Here's how the part is built. I have some questions about the finished solid (model axes, mm). A direction names the side the tool comes from. Coordinates: 2 decimals unless noted, no trailing zeros. Write each loop counter-clockwise with the first axis right and the second up, starting at its lowest first coordinate (ties: lowest second). Pieces come first, ordered by that corner, then holes. Notation, with made-up numbers: (34.5, 74.5) -> (77.5, 74.5) arc R17 cw to (77.5, 96.5) -> close; hole circle Ø2 at (67, -6). An arc over 180 degrees is marked (long way). Answer in a Markdown table with one row per item. Add a question column.
from build123d import *

# Parameters (mm, degrees)
F1_DEPTH  = 3.81
F4_DEPTH  = 71.628
F6_DEPTH  = 1.27
F7_W      = 13.462
F7_H      = 6.477
F8_DEPTH  = 25.4
F9_W      = 54.61
F9_H      = 4.318
F10_DEPTH = 25.4


with BuildPart() as f1:
    # F0 (on Front) → F1 (new body)
    with BuildSketch(Plane.XZ):
        Polygon((-38.4448663006, 16.8945933835), (-38.4448663006, 14.7355933835), (33.1831336994, 14.7355933835), (33.1831336994, 16.8945933835), (28.6111336994, 16.8945933835), (27.0871336994, 16.8945933835), (22.5151336994, 16.8945933835), (20.9911336994, 16.8945933835), (16.4191336994, 16.8945933835), (14.8951336994, 16.8945933835), (10.3231336994, 16.8945933835), (8.7991336994, 16.8945933835), (4.2271336994, 16.8945933835), (2.7031336994, 16.8945933835), (-1.8688663006, 16.8945933835), (-3.3928663006, 16.8945933835), (-7.9648663006, 16.8945933835), (-9.4888663006, 16.8945933835), (-14.0608663006, 16.8945933835), (-15.5848663006, 16.8945933835), (-20.1568663006, 16.8945933835), (-21.6808663006, 16.8945933835), (-26.2528663006, 16.8945933835), (-27.7768663006, 16.8945933835), (-32.3488663006, 16.8945933835), (-33.8728663006, 16.8945933835), align=None)
        Polygon((-37.1748663006, 21.2125933835), (-38.4448663006, 16.8945933835), (-33.8728663006, 16.8945933835), (-35.1428663006, 21.2125933835), align=None)
        Polygon((28.6111336994, 16.8945933835), (33.1831336994, 16.8945933835), (31.9131336994, 21.2125933835), (29.8811336994, 21.2125933835), align=None)
        Polygon((-31.0788663006, 21.2125933835), (-32.3488663006, 16.8945933835), (-27.7768663006, 16.8945933835), (-29.0468663006, 21.2125933835), align=None)
        Polygon((22.5151336994, 16.8945933835), (27.0871336994, 16.8945933835), (25.8171336994, 21.2125933835), (23.7851336994, 21.2125933835), align=None)
        Polygon((-24.9828663006, 21.2125933835), (-26.2528663006, 16.8945933835), (-21.6808663006, 16.8945933835), (-22.9508663006, 21.2125933835), align=None)
        Polygon((16.4191336994, 16.8945933835), (20.9911336994, 16.8945933835), (19.7211336994, 21.2125933835), (17.6891336994, 21.2125933835), align=None)
        Polygon((-18.8868663006, 21.2125933835), (-20.1568663006, 16.8945933835), (-15.5848663006, 16.8945933835), (-16.8548663006, 21.2125933835), align=None)
        Polygon((10.3231336994, 16.8945933835), (14.8951336994, 16.8945933835), (13.6251336994, 21.2125933835), (11.5931336994, 21.2125933835), align=None)
        Polygon((-12.7908663006, 21.2125933835), (-14.0608663006, 16.8945933835), (-9.4888663006, 16.8945933835), (-10.7588663006, 21.2125933835), align=None)
        Polygon((4.2271336994, 16.8945933835), (8.7991336994, 16.8945933835), (7.5291336994, 21.2125933835), (5.4971336994, 21.2125933835), align=None)
        Polygon((-6.6948663006, 21.2125933835), (-7.9648663006, 16.8945933835), (-3.3928663006, 16.8945933835), (-4.6628663006, 21.2125933835), align=None)
        Polygon((-1.8688663006, 16.8945933835), (2.7031336994, 16.8945933835), (1.4331336994, 21.2125933835), (-0.5988663006, 21.2125933835), align=None)
    extrude(amount=F1_DEPTH)

    # F3 (on plane+point) → F4 (join, through all)
    with BuildSketch(Plane.YZ.offset(33.1831336994)):
        Polygon((-13.97, 14.7355933835), (-3.81, 14.7355933835), (-3.81, 16.8945933835), (-10.16, 16.8945933835), (-10.16, 19.0535933835), (-13.97, 19.0535933835), (-13.97, 16.8945933835), align=None)
    extrude(amount=-F4_DEPTH)

    # F5 (on face) → F6 (join)
    with BuildSketch(Plane(origin=(0, 0, 0), x_dir=(-1, 0, 0), z_dir=(0, 1, 0))):
        Polygon((33.8728663006, 16.8945933835), (35.1428663006, 21.2125933835), (31.0788663006, 21.2125933835), (32.3488663006, 16.8945933835), align=None)
        Polygon((27.7768663006, 16.8945933835), (29.0468663006, 21.2125933835), (24.9828663006, 21.2125933835), (26.2528663006, 16.8945933835), align=None)
        Polygon((21.6808663006, 16.8945933835), (22.9508663006, 21.2125933835), (18.8868663006, 21.2125933835), (20.1568663006, 16.8945933835), align=None)
        Polygon((15.5848663006, 16.8945933835), (16.8548663006, 21.2125933835), (12.7908663006, 21.2125933835), (14.0608663006, 16.8945933835), align=None)
        Polygon((9.4888663006, 16.8945933835), (10.7588663006, 21.2125933835), (6.6948663006, 21.2125933835), (7.9648663006, 16.8945933835), align=None)
        Polygon((3.3928663006, 16.8945933835), (4.6628663006, 21.2125933835), (0.5988663006, 21.2125933835), (1.8688663006, 16.8945933835), align=None)
        Polygon((-1.4331336994, 21.2125933835), (-5.4971336994, 21.2125933835), (-4.2271336994, 16.8945933835), (-2.7031336994, 16.8945933835), align=None)
        Polygon((-7.5291336994, 21.2125933835), (-11.5931336994, 21.2125933835), (-10.3231336994, 16.8945933835), (-8.7991336994, 16.8945933835), align=None)
        Polygon((-13.6251336994, 21.2125933835), (-17.6891336994, 21.2125933835), (-16.4191336994, 16.8945933835), (-14.8951336994, 16.8945933835), align=None)
        Polygon((-19.7211336994, 21.2125933835), (-23.7851336994, 21.2125933835), (-22.5151336994, 16.8945933835), (-20.9911336994, 16.8945933835), align=None)
        Polygon((-25.8171336994, 21.2125933835), (-29.8811336994, 21.2125933835), (-28.6111336994, 16.8945933835), (-27.0871336994, 16.8945933835), align=None)
        Polygon((-33.1831336994, 14.7355933835), (38.4448663006, 14.7355933835), (38.4448663006, 16.8945933835), (37.1748663006, 21.2125933835), (35.1428663006, 21.2125933835), (33.8728663006, 16.8945933835), (32.3488663006, 16.8945933835), (31.0788663006, 21.2125933835), (29.0468663006, 21.2125933835), (27.7768663006, 16.8945933835), (26.2528663006, 16.8945933835), (24.9828663006, 21.2125933835), (22.9508663006, 21.2125933835), (21.6808663006, 16.8945933835), (20.1568663006, 16.8945933835), (18.8868663006, 21.2125933835), (16.8548663006, 21.2125933835), (15.5848663006, 16.8945933835), (14.0608663006, 16.8945933835), (12.7908663006, 21.2125933835), (10.7588663006, 21.2125933835), (9.4888663006, 16.8945933835), (7.9648663006, 16.8945933835), (6.6948663006, 21.2125933835), (4.6628663006, 21.2125933835), (3.3928663006, 16.8945933835), (1.8688663006, 16.8945933835), (0.5988663006, 21.2125933835), (-1.4331336994, 21.2125933835), (-2.7031336994, 16.8945933835), (-4.2271336994, 16.8945933835), (-5.4971336994, 21.2125933835), (-7.5291336994, 21.2125933835), (-8.7991336994, 16.8945933835), (-10.3231336994, 16.8945933835), (-11.5931336994, 21.2125933835), (-13.6251336994, 21.2125933835), (-14.8951336994, 16.8945933835), (-16.4191336994, 16.8945933835), (-17.6891336994, 21.2125933835), (-19.7211336994, 21.2125933835), (-20.9911336994, 16.8945933835), (-22.5151336994, 16.8945933835), (-23.7851336994, 21.2125933835), (-25.8171336994, 21.2125933835), (-27.0871336994, 16.8945933835), (-28.6111336994, 16.8945933835), (-29.8811336994, 21.2125933835), (-31.9131336994, 21.2125933835), (-33.1831336994, 16.8945933835), align=None)
        Polygon((37.1748663006, 21.2125933835), (38.4448663006, 16.8945933835), (38.4448663006, 21.2125933835), align=None)
    extrude(amount=F6_DEPTH)

    # F7 (on face) → F8 (join)
    with BuildSketch(Plane(origin=(0, 1.27, 0), x_dir=(-1, 0, 0), z_dir=(0, 1, 0))):
        with Locations((31.7138663006, 17.9740933835)):
            Rectangle(F7_W, F7_H)
    extrude(amount=F8_DEPTH)

    # F9 (on face) → F10 (cut)
    with BuildSketch(Plane.XY.offset(16.8945933835)):
        with Locations((-2.6308663007, -6.985)):
            Rectangle(F9_W, F9_H)
        with BuildLine():
            Line((24.6741336994, -4.826), (24.6741336994, -9.144))
            ThreePointArc((24.6741336994, -9.144), (26.8331336994, -6.985), (24.6741336994, -4.826))
        make_face()
        with BuildLine():
            ThreePointArc((-29.9358663007, -4.826), (-32.0948663007, -6.985), (-29.9358663007, -9.144))
            Line((-29.9358663007, -9.144), (-29.9358663007, -4.826))
        make_face()
    extrude(amount=-F10_DEPTH, mode=Mode.SUBTRACT)


solid = f1.part
Q1. For faces 3 (the flat face through (-28.4, -1.88, 19.02)), 4 (the flat face through (-3, -4.826, 16)), 5 (the flat face through (5, 1.27, 18)), which set-ups out of +Z, -Z, +X, -X, +Y, -Y let a thin tool reach every point of the face, with its end or its side?
Q2. Imagine slicing it at D-D on y = 11. Please give me the cut outline in (x, z), plus the area to 3 significant figures.
Q3. Imagine slicing it at C-C on y = -5.5. Please give me the cut outline in (x, z).
Q4. I'm going to push flat-ended pins straight in: P1, Ø1, axis at x = -10, z = 17.5, coming from the +Y side; P2, Ø1.9, axis at x = -6.5, y = -13, coming from the +Z side; P3, Ø3, axis at y = 10.5, z = 18.5, coming from the +X side; P4, Ø1, axis at x = -15.5, y = 3, coming from the -Z side. Where does each tip first touch, or does it pass through?
Q5. If we mould it in two halves opening along X, with no side actions, what happens to faces 1 (the flat face through (-7.321, -1.878, 19.084)), 2 (the flat face through (6, -3.81, 19))? For each: pulls with the +X half, pulls with the -X half, needs draft (parallel to the pull), parting line crosses it, or undercut.
Q6. I need wall thicknesses on line 1 (Y direction, x = -25.5, z = 15); line 2 (Y direction, x = 12.5, z = 17.5); line 3 (Y direction, x = 9, z = 20.5). Which ranges of each line are inside material? Lowest first, please. Write a range as [from, to].
Q7. Imagine slicing it at B-B on x = -6. Please give me the cut outline in (y, z), plus the area to 3 significant figures.
Q8. Imagine slicing it at A-A on z = 16. Please give me the cut outline in (x, y) (3 decimals), plus the area to 3 significant figures.
Result sheet:
| question | item | result |
|---|---|---|
| 1 | face 3 | +Z |
| 1 | face 4 | +Z, -Z |
| 1 | face 5 | +Z, -Z, +X, +Y |
| 2 | outline | (-38.44, 14.74) -> (-24.98, 14.74) -> (-24.98, 21.21) -> (-38.44, 21.21) -> close |
| 2 | area | 87.2 mm^2 |
| 3 | outline | (-38.44, 14.74) -> (-31.5, 14.74) -> (-31.5, 16.89) -> (-38.44, 16.89) -> close; (26.24, 14.74) -> (33.18, 14.74) -> (33.18, 16.89) -> (26.24, 16.89) -> close |
| 4 | P1 | stops at y = 1.27 |
| 4 | P2 | stops at z = 19.05 |
| 4 | P3 | stops at x = -24.98 |
| 4 | P4 | passes through |
| 5 | face 1 | undercut |
| 5 | face 2 | needs draft |
| 6 | line 1 | y = [-13.97, -9.14], [-4.83, 26.67] |
| 6 | line 2 | y = [-13.97, -10.16], [-3.81, 1.27] |
| 6 | line 3 | y = [0, 1.27] |
| 7 | outline | (-13.97, 14.74) -> (-9.14, 14.74) -> (-9.14, 16.89) -> (-10.16, 16.89) -> (-10.16, 19.05) -> (-13.97, 19.05) -> close; (-4.83, 14.74) -> (1.27, 14.74) -> (1.27, 21.21) -> (-3.81, 21.21) -> (-3.81, 16.89) -> (-4.83, 16.89) -> close |
| 7 | area | 53.7 mm^2 |
| 8 | outline | (-38.445, -13.97) -> (33.183, -13.97) -> (33.183, 1.27) -> (-24.983, 1.27) -> (-24.983, 26.67) -> (-38.445, 26.67) -> close; hole (-29.936, -9.144) -> (24.674, -9.144) arc R2.159 ccw to (24.674, -4.826) -> (-29.936, -4.826) arc R2.159 ccw to start |
| 8 | area | 1,180 mm^2 |
